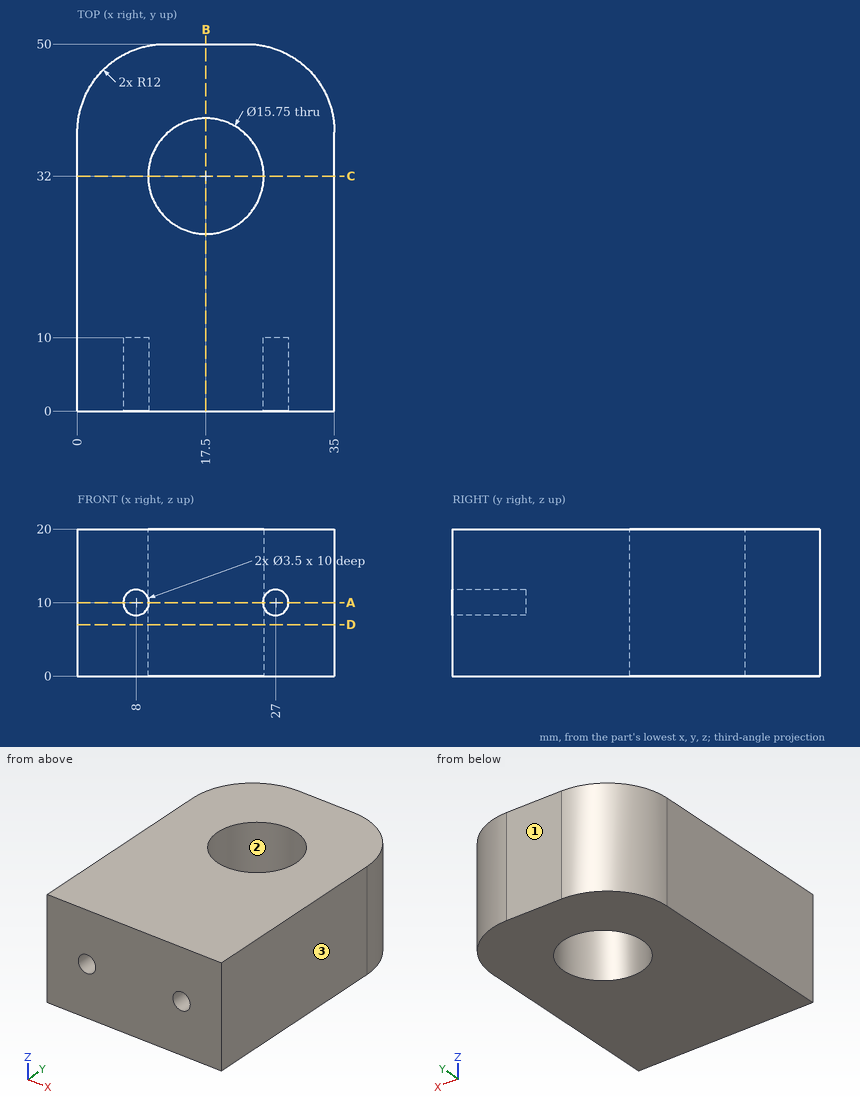
Here's the drawing with two shaded views (mm, measured from the low corner). I have some questions. Coordinates: 2 decimals unless noted, no trailing zeros. Order: outer loops, then holes, each group sorted by start corner. A loop starts at its lowest first (then second) coordinate and runs counter-clockwise, first axis right, second up.
Item 1: If we section it at B-B, the plane x = 17.5: List the corners of the cut face in (y, z) for me (3 decimals).
Response values:
outline: (0, 0) - (24.125, 0) - (24.125, 20) - (0, 20) - close; (39.875, 0) - (50, 0) - (50, 20) - (39.875, 20) - close
Item 2: If we section it at C-C, the plane y = 32: List the corners of the cut face in (x, z) for me (3 decimals), then the cut area to 3 significant figures.
Response values:
outline: (0, 0) - (9.625, 0) - (9.625, 20) - (0, 20) - close; (25.375, 0) - (35, 0) - (35, 20) - (25.375, 20) - close
area: 385 mm2
Item 3: If we section it at A-A, the plane z = 10: List the corners of the cut face in (x, y) for me (3 decimals), then the cut area to 3 significant figures.
Response values:
outline: (0, 0) - (6.25, 0) - (6.25, 10) - (9.75, 10) - (9.75, 0) - (25.25, 0) - (25.25, 10) - (28.75, 10) - (28.75, 0) - (35, 0) - (35, 38) arc R12 ccw to (23, 50) - (12, 50) arc R12 ccw to (0, 38) - close; hole circle Ø15.75 at (17.5, 32)
area: 1,420 mm2
Item 4: Thinking about a two-plate mould opening in X: for the marked faces 1, 2 and 3, which applies, pulls with the +X half, pulls with the -X half, needs draft (parallel to the pull), parting line crosses it, or undercut?
Response values:
face 1: needs draft
face 2: undercut
face 3: pulls with the +X half
Item 5: I'm going to push flat-ended pins straight in: pin 1 Ø1.8 at (x, z) = (27.5, 10.5) entering from -Y; pin 2 Ø4 at (x, z) = (27, 10) entering from +Y; pin 3 Ø2 at (x, z) = (8, 10) entering from +Y. Where does each tip first touch, or does it pass through?
Response values:
pin 1: stops at y = 10
pin 2: stops at y = 49.83
pin 3: stops at y = 49.62
Item 6: If we section it at D-D, the plane z = 7: List the corners of the cut face in (x, y) for me (3 decimals).
Response values:
outline: (0, 0) - (35, 0) - (35, 38) arc R12 ccw to (23, 50) - (12, 50) arc R12 ccw to (0, 38) - close; hole circle Ø15.75 at (17.5, 32)
Item 7: I need wall thicknesses on probe 1 along Y at (x, z) = (17.5, 8.25) (3 decimals); probe 2 along Z at (x, y) = (27, 2.75); probe 3 along Y at (x, z) = (23, 3). Which ranges of each line are inside material? Lowest first, please.
Response values:
probe 1: y = 0 to 24.125, 39.875 to 50
probe 2: z = 0 to 8.25, 11.75 to 20
probe 3: y = 0 to 26.36, 37.64 to 50
